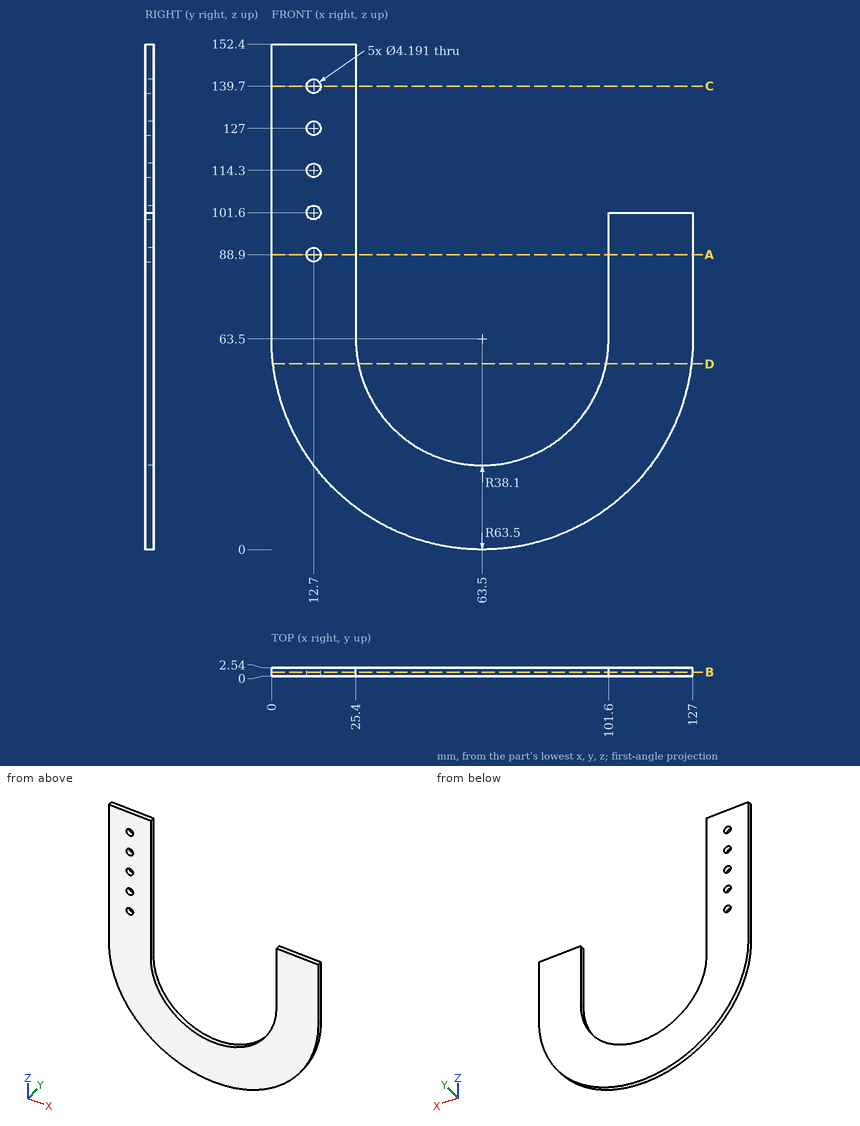
The drawing under review shows one solid part. Ordinate dimensions are in mm from its lowest x, y, z. Round coordinates to 2 decimals unless told otherwise and drop trailing zeros. Write each loop counter-clockwise with the first axis right and the second up, starting at its lowest first coordinate (ties: lowest second). Pieces come first, ordered by that corner, then holes. Notation, with made-up numbers: (59, -33) - (67, -33) arc R36 ccw to (67, 6) - close; hole circle Ø3 at (22.25, 29). An arc over 180 degrees is marked (long way). Put each result on its own line as item: value.
Q1. We need section A-A (z = 88.9). Give the boundary of the cut face in (x, y).
Solved:
outline: (0, 0) - (10.6, 0) - (10.6, 2.54) - (0, 2.54) - close; (14.8, 0) - (25.4, 0) - (25.4, 2.54) - (14.8, 2.54) - close; (101.6, 0) - (127, 0) - (127, 2.54) - (101.6, 2.54) - close
Q2. We need section D-D (z = 56). Give the boundary of the cut face in (x, y), and give its area (3 significant figures).
Solved:
outline: (0.44, 0) - (26.15, 0) - (26.15, 2.54) - (0.44, 2.54) - close; (100.85, 0) - (126.56, 0) - (126.56, 2.54) - (100.85, 2.54) - close
area: 131 mm2
Q3. Wall thickness on probe 1 along X at (y, z) = (1.6, 88.9); probe 2 along X at (y, z) = (0.3, 81); probe 3 along X at (y, z) = (1.8, 139.7): over which ranges is each line inside the solid? List them lowest first.
Solved:
probe 1: x = 0 to 10.6, 14.8 to 25.4, 101.6 to 127
probe 2: x = 0 to 25.4, 101.6 to 127
probe 3: x = 0 to 10.6, 14.8 to 25.4
Q4. We need section B-B (y = 1.15). Give the boundary of the cut face in (x, z).
Solved:
outline: (0, 63.5) arc R63.5 ccw to (127, 63.5) - (127, 101.6) - (101.6, 101.6) - (101.6, 63.5) arc R38.1 cw to (25.4, 63.5) - (25.4, 152.4) - (0, 152.4) - close; hole circle Ø4.19 at (12.7, 88.9); hole circle Ø4.19 at (12.7, 101.6); hole circle Ø4.19 at (12.7, 114.3); hole circle Ø4.19 at (12.7, 127); hole circle Ø4.19 at (12.7, 139.7)
Q5. Insertion check: pin 1 Ø4 at (x, z) = (12.7, 114.3) entering from -Y; pin 2 Ø1 at (x, y) = (22.5, 1) entering from -Z; pin 3 Ø1 at (x, y) = (46.5, 1) entering from -Z. Each pin has a flat end and moves straight along its axis. Give the tip position at first contact, or say it passes through.
Solved:
pin 1: passes through
pin 2: stops at z = 14.59
pin 3: stops at z = 2.18
Q6. We need section C-C (z = 139.7). Give the boundary of the cut face in (x, y).
Solved:
outline: (0, 0) - (10.6, 0) - (10.6, 2.54) - (0, 2.54) - close; (14.8, 0) - (25.4, 0) - (25.4, 2.54) - (14.8, 2.54) - close
